Autodesk Inventor part; units mm, degrees
ref_plane "YZ Plane" through (0, 0, 0) normal (1, 0, 0) x (0, 1, 0)
ref_plane "XZ Plane" through (0, 0, 0) normal (0, 1, 0) x (-1, 0, 0)
ref_plane "XY Plane" through (0, 0, 0) normal (0, 0, 1) x (1, 0, 0)
sketch "スケッチ1" plane through (0, 0, 0) normal (0, 0, 1) x (1, 0, 0)
  line L0 (0, 0) -> (112, 0)
  line L1 (112, 0) -> (112, -75)
  line L2 (112, -75) -> (0, -75)
  line L3 (0, -75) -> (0, 0)
  dimension "d0" = 112
  dimension "d1" = 75
extrude "押し出し1" add sketch "スケッチ1" along normal blind 5.5
sketch "スケッチ2" plane through (0, 0, 5.5) normal (0, 0, 1) x (1, 0, 0)
  line L0 (112, 0) -> (0, 0)
  line L1 (0, 0) -> (0, -75)
  line L2 (0, -75) -> (112, -75)
  point P0 (7.5, -7.5)
  point P1 (107.5, -7.5)
  point P2 (107.5, -67.5)
  point P3 (7.5, -67.5)
  dimension "d4" = 7.5
  dimension "d5" = 7.5
  dimension "d6" = 7.5
  dimension "d7" = 100
  dimension "d8" = 60
  dimension "d9" = 60
  dimension "d10" = 100
  dimension "d19" = 7.5
  dimension "d51" = 7.5
hole "穴1" at (7.5, -7.5, 5.5) at (107.5, -7.5, 5.5) at (107.5, -67.5, 5.5) at (7.5, -67.5, 5.5) direction (0, 0, -1) diameter 3 end through all
fillet "フィレット1" radius 6 4 edges at (112, 0, 2.75) (112, -75, 2.75) (0, 0, 2.75) (0, -75, 2.75)
sketch "スケッチ3" plane through (0, 0, 0) normal (0, 0, -1) x (-1, 0, 0)
  circle A0 centre (-42, -45) radius 15.5
  line L0 (-112, -69) -> (-112, -6)
  line L1 (0, -6) -> (0, -69)
  line L2 (-106, 0) -> (-6, 0)
  line L3 (-6, -75) -> (-106, -75)
  line L4 (-42, -45) -> (-26.5, -45)
  line L5 (-42, -45) -> (-49.75, -31.5766)
  line L6 (-42, -45) -> (-49.75, -58.4234)
  point P0 (0, 0)
  dimension "d20" = 31
  dimension "d21" = 70
  dimension "d22" = 112
  dimension "d23" = 75
  dimension "d24" = 30
  dimension "d25" = 120
  dimension "d26" = 120
hole "穴2" at (49.75, -58.4234, 0) at (49.75, -31.5766, 0) at (26.5, -45, 0) direction (0, 0, 1) diameter 3 end through all
sketch "スケッチ4" plane through (0, 0, 0) normal (0, 0, -1) x (-1, 0, 0)
  line L0 (-42, -45) -> (-42, -38)
  line L1 (-6, -75) -> (-106, -75)
  line L2 (-106, 0) -> (-6, 0)
  line L3 (-112, -69) -> (-112, -6)
  point P0 (0, 0)
  dimension "d34" = 7
  dimension "d35" = 30
  dimension "d36" = 75
  dimension "d37" = 70
hole "穴3" at (42, -38, 0) direction (0, 0, 1) diameter 12 end through all
sketch "スケッチ5" plane through (0, 0, 5.5) normal (0, 0, 1) x (1, 0, 0)
  circle A0 centre (72, -38) radius 4
  circle A1 centre (42, -38) radius 6
  line L0 (106, 0) -> (6, 0)
  point P0 (0, 0)
  dimension "d45" = 8
  dimension "d46" = 30
  dimension "d47" = 38
  dimension "d48" = 38
extrude "押し出し2" cut sketch "スケッチ5" against normal through all contours A0
equation "\"d48\" = d47"
properties part number "前後直動12x12_4" material "木材 (カエデ材)"
Verification items for the finished model (mm, model axes). Round coordinates to 2 decimals unless told otherwise and drop trailing zeros. Write each loop counter-clockwise with the first axis right and the second up, starting at its lowest first coordinate (ties: lowest second). Pieces come first, ordered by that corner, then holes.
(1) Section check B-B (x = 26.5). Enter the section's corners in (y, z), plus the area to 3 significant figures.
Returned:
outline: (-75, 0) - (-46.5, 0) - (-46.5, 5.5) - (-75, 5.5) - close; (-43.5, 0) - (0, 0) - (0, 5.5) - (-43.5, 5.5) - close
area: 396 mm2
(2) Section check D-D (x = 49.75). Enter the section's corners in (y, z).
Returned:
outline: (-75, 0) - (-59.92, 0) - (-59.92, 5.5) - (-75, 5.5) - close; (-56.92, 0) - (-33.08, 0) - (-33.08, 5.5) - (-56.92, 5.5) - close; (-30.08, 0) - (0, 0) - (0, 5.5) - (-30.08, 5.5) - close
(3) Section check A-A (y = -7.5). Enter the section's corners in (x, z).
Returned:
outline: (0, 0) - (6, 0) - (6, 5.5) - (0, 5.5) - close; (9, 0) - (106, 0) - (106, 5.5) - (9, 5.5) - close; (109, 0) - (112, 0) - (112, 5.5) - (109, 5.5) - close
(4) Material ranges on line 1 (X direction, y = -7.5, z = 3.7); line 2 (X direction, y = -45, z = 1.85); line 3 (Y direction, x = 49.75, z = 3.35), recorded low to high.
Returned:
line 1: x = 0 to 6, 9 to 106, 109 to 112
line 2: x = 0 to 25, 28 to 112
line 3: y = -75 to -59.92, -56.92 to -33.08, -30.08 to 0
(5) Section check C-C (z = 1.8). Give the number of separate pieces and of enclosed holes in the cut face, plus the area to 3 significant figures.
Returned:
separate pieces: 1
enclosed holes: 9
area: 8,160 mm2
(6) Depth check by flat-ended pin: pin 1 Ø1.8 at (x, y) = (107.5, -67.5) entering from -Z. Enter the tip coordinate at first touch or a pass-through.
Returned:
pin 1: passes through
(7) Mould release check, pull along Y, two halves, no side actions. Record for faces 1 (the flat face through (0, -38, 3)), 2 (the cylindrical face through (71.479, -34.034, 2.788)), 3 (the cylindrical face through (110.196, -73.289, 2.788)): pulls with the +Y half, pulls with the -Y half, needs draft (parallel to the pull), parting line crosses it, or undercut.
Returned:
face 1: needs draft
face 2: undercut
face 3: pulls with the -Y half
